Could you check a few things on this model? Use its own coordinates, in mm. A direction names the side the tool comes from. Round coordinates to 2 decimals unless told otherwise and drop trailing zeros. Write each loop counter-clockwise with the first axis right and the second up, starting at its lowest first coordinate (ties: lowest second). Pieces come first, ordered by that corner, then holes. Notation, with made-up numbers: (13, 67.25) -> (46, 67.25) arc R22 ccw to (46, 93.25) -> close; hole circle Ø11 at (87.25, 3). An arc over 180 degrees is marked (long way). Answer in a Markdown table with one row per item.
from build123d import *

# Parameters (mm, degrees)
SKETCH_W        = 4.72
SKETCH_H        = 5.2
PAD_DEPTH       = 18.3
SKETCH001_W     = 29
SKETCH001_H     = 11.3
POCKET_DEPTH    = 38.001
POCKET005_DEPTH = 15.3
SKETCH003_R     = 1.5
POCKET006_DEPTH = 5
FILLET_R        = 1
FILLET001_R     = 1
FILLET002_R     = 1
FILLET003_R     = 1
FILLET004_R     = 1


with BuildPart() as part:
    # Sketch → Pad (new body)
    with BuildSketch(Plane.XY):
        Polygon((-19, 19), (-19, -19), (19, -19), (19, 19), (17, 19), (17, 26.7), (6, 26.7), (6, 19), (-6, 19), (-6, 26.7), (-17, 26.7), (-17, 19), align=None)
        with Locations((-12.41, 21.6)):
            Rectangle(SKETCH_W, SKETCH_H, mode=Mode.SUBTRACT)
        with Locations((12.41, 21.6)):
            Rectangle(SKETCH_W, SKETCH_H, mode=Mode.SUBTRACT)
    extrude(amount=PAD_DEPTH)

    # Sketch001 (on Face3 of Pad) → Pocket (cut, through all)
    with BuildSketch(Plane.YZ.offset(19)):
        with Locations((12.2, 5.65)):
            Rectangle(SKETCH001_W, SKETCH001_H)
    extrude(amount=-POCKET_DEPTH, mode=Mode.SUBTRACT)

    # Sketch002 (on Face6 of Pocket) → Pocket005 (cut)
    with BuildSketch(Plane.XY.offset(18.3)):
        Polygon((-9.25, -19), (9.25, -19), (9.25, 6.35), (6, 6.35), (6, 19), (-6, 19), (-6, 6.35), (-9.25, 6.35), align=None)
    extrude(amount=-POCKET005_DEPTH, mode=Mode.SUBTRACT)

    # Sketch003 → Pocket006 (cut)
    with BuildSketch(Plane.XY.offset(4)):
        with Locations((-5.25, -5.15)):
            Circle(SKETCH003_R)
        with Locations((5.25, -5.15)):
            Circle(SKETCH003_R)
    extrude(amount=-POCKET006_DEPTH, mode=Mode.SUBTRACT)

    # Fillet
    fillet_edges = [part.edges().sort_by_distance(p)[0] for p in [
        (19, 19, 14.8),
        (17, 26.7, 14.8),
        (6, 26.7, 14.8),
        (-6, 26.7, 14.8),
        (-17, 26.7, 14.8),
        (-19, 19, 14.8),
    ]]
    fillet(fillet_edges, radius=FILLET_R)

    # Fillet001
    fillet001_edges = [part.edges().sort_by_distance(p)[0] for p in [
        (19, -10.65, 0),
        (-19, -10.65, 0),
    ]]
    fillet(fillet001_edges, radius=FILLET001_R)

    # Fillet002
    fillet002_edges = [part.edges().sort_by_distance(p)[0] for p in [
        (14.125, -2.3, 11.3),
        (-14.125, -2.3, 11.3),
    ]]
    fillet(fillet002_edges, radius=FILLET002_R)

    # Fillet003
    fillet003_edges = [part.edges().sort_by_distance(p)[0] for p in [
        (0, -2.3, 0),
    ]]
    fillet(fillet003_edges, radius=FILLET003_R)

    # Fillet004
    fillet004_edges = [part.edges().sort_by_distance(p)[0] for p in [
        (0, -19, 0),
        (19, -19, 9.65),
        (-19, -19, 9.65),
        (-14.125, -19, 18.3),
        (14.125, -19, 18.3),
    ]]
    fillet(fillet004_edges, radius=FILLET004_R)


solid = part.part
1) For pin 1 (10 mm diameter, centred on x = 4, z = 6.5, fed in from +Y); pin 2 (1.6 mm diameter, centred on x = 8, z = 15.5, fed in from -Y); pin 3 (5.5 mm diameter, centred on y = 22.5, z = 14, fed in from +X), each with a flat end and sliding along its axis, tell me the tip position at first contact or that it passes through.
Findings:
| item | result |
|---|---|
| pin 1 | stops at y = -2.3 |
| pin 2 | stops at y = 6.35 |
| pin 3 | stops at x = 17 |
2) Please list where these lines run through material, in increasing order: line 1 (Y direction, x = 5.25, z = 1.2); line 2 (Y direction, x = 10.5, z = 17); line 3 (X direction, y = -5, z = 10).
Findings:
| item | result |
|---|---|
| line 1 | y = -19 to -6.65, -3.65 to -2.3 |
| line 2 | y = -19 to 19, 24.2 to 26.7 |
| line 3 | x = -19 to -9.25, 9.25 to 19 |
3) Imagine slicing it at A-A, the plane z = 13.75. Count the separate pieces of the cut face and the enclosed holes in it, plus the area to 3 significant figures.
Findings:
| item | result |
|---|---|
| separate pieces | 2 |
| enclosed holes | 2 |
| area | 942 mm^2 |
4) For faces 1 (the face through (8, 6.35, 15)), 2 (the face through (9.25, -9, 11)), 3 (the face through (17.5, 19, 15.3)), 4 (the face through (-6.301, 26.415, 14.849)), 5 (the face through (14.77, 22, 15)), which set-ups out of +Z, -Z, +X, -X, +Y, -Y let a thin tool reach every point of the face, with its end or its side?
Findings:
| item | result |
|---|---|
| face 1 | +Z, -Z, -Y |
| face 2 | +Z, -Y |
| face 3 | +Z, -Z, +X, +Y |
| face 4 | +Z, -Z, +Y |
| face 5 | +Z, -Z |
5) Imagine slicing it at C-C, the plane y = -5.15. Please give me the cut outline in (x, z).
Findings:
| item | result |
|---|---|
| outline | (-19, 1) arc R1 ccw to (-18, 0) -> (-6.75, 0) -> (-6.75, 3) -> (-9.25, 3) -> (-9.25, 18.3) -> (-19, 18.3) -> close; (-3.75, 0) -> (3.75, 0) -> (3.75, 3) -> (-3.75, 3) -> close; (6.75, 0) -> (18, 0) arc R1 ccw to (19, 1) -> (19, 18.3) -> (9.25, 18.3) -> (9.25, 3) -> (6.75, 3) -> close |
6) Imagine slicing it at B-B, the plane x = -5.25. Please give me the cut outline in (y, z), plus the area to 3 significant figures.
Findings:
| item | result |
|---|---|
| outline | (-19, 1) arc R1 ccw to (-18, 0) -> (-6.65, 0) -> (-6.65, 3) -> (-19, 3) -> close; (-3.65, 0) -> (-3.3, 0) arc R1 ccw to (-2.3, 1) -> (-2.3, 3) -> (-3.65, 3) -> close |
| area | 40.7 mm^2 |
7) Imagine slicing it at D-D, the plane z = 6.25. Please give me the cut outline in (x, y), plus the area to 3 significant figures.
Findings:
| item | result |
|---|---|
| outline | (-19, -18) arc R1 ccw to (-18, -19) -> (-9.25, -19) -> (-9.25, -2.3) -> (-18, -2.3) arc R1 ccw to (-19, -3.3) -> close; (9.25, -19) -> (18, -19) arc R1 ccw to (19, -18) -> (19, -3.3) arc R1 ccw to (18, -2.3) -> (9.25, -2.3) -> close |
| area | 325 mm^2 |
8) Thinking about a two-plate mould opening in X: for faces 6 (the face through (-10.05, 22, 15)), 7 (the face through (-12, 13, 11.3)), 8 (the face through (-16.715, 26.399, 14.849)), which applies, +X half, -X half, draft (parallel to the pull), parting line (faces both ways), or undercut?
Findings:
| item | result |
|---|---|
| face 6 | undercut |
| face 7 | draft |
| face 8 | -X half |
